from build123d import *

# Parameters (mm, degrees)
RESSALTO_EXTRUS_O1_DEPTH = 20


with BuildPart() as part:
    # Esboço1 → Ressalto-extrusão1 (new body, symmetric)
    with BuildSketch(Plane.XY):
        with BuildLine():
            Line((-40, 0), (40, 0))
            ThreePointArc((40, 0), (47.071067812, 2.928932188), (50, 10))
            Line((50, 10), (50, 110))
            ThreePointArc((50, 110), (51.339745962, 115), (55, 118.660254038))
            Line((55, 118.660254038), (95, 141.754264805))
            ThreePointArc((95, 141.754264805), (98.660254038, 145.414518843), (100, 150.414518843))
            Line((100, 150.414518843), (100, 290))
            ThreePointArc((100, 290), (97.071067812, 297.071067812), (90, 300))
            Line((90, 300), (-90, 300))
            ThreePointArc((-90, 300), (-97.071067812, 297.071067812), (-100, 290))
            Line((-100, 290), (-100, 150.414518843))
            ThreePointArc((-100, 150.414518843), (-98.660254038, 145.414518843), (-95, 141.754264805))
            Line((-95, 141.754264805), (-55, 118.660254038))
            ThreePointArc((-55, 118.660254038), (-51.339745962, 115), (-50, 110))
            Line((-50, 110), (-50, 10))
            ThreePointArc((-50, 10), (-47.071067812, 2.928932188), (-40, 0))
        make_face()
    extrude(amount=RESSALTO_EXTRUS_O1_DEPTH, both=True)


solid = part.part
Could you check a few things on this model? Use its own coordinates, in mm. A direction names the side the tool comes from. Give positions to 0.01 mm unless a question says otherwise; leave off trailing zeros. Order: outer loops, then holes, each group sorted by start corner. A loop starts at its lowest first (then second) coordinate and runs counter-clockwise, first axis right, second up. Notation, with made-up numbers: (-10, 30.5) - (-2, 30.5) arc R28 ccw to (-2, 66.5) - close; hole circle Ø1 at (43, -17.75). An arc over 180 degrees is marked (long way). Return JSON: item names as keys, results as strings. Group by question number.
Q1. Will these pins go through, and if not, where does the flat tip stop? pin 1 Ø8 at (x, z) = (-61.5, -15.5) entering from -Y; pin 2 Ø12 at (y, z) = (40, 9) entering from +X.
Q2. Suppose I cut it at C-C, the plane x = -79. Please give me the cut outline in (y, z).
Q3. Which directions (+Z, -Z, +X, -X, +Y, -Y) give clear straight access to the entire face, cutting with the end or side of a thin tool? Please do faces 1 (the face through (-50, 61, 0)), 2 (the face through (50, 59, 0)), 3 (the face through (-1, 0, 0)).
Q4. Suppose I cut it at B-B, the plane y = 69. Please give me the cut outline in (x, z).
Q5. Please list where these lines run through material, in increasing order: line 1 along X through (y, z) = (18, -8); line 2 along Y through (x, z) = (58.5, 6); line 3 along Y through (x, z) = (57, 6). Write a range as [from, to].
Q6. Suppose I cut it at A-A, the plane z = 4. Please give me the cut outline in (x, y), and give its area (3 significant figures).
Resolved:
{
 "1": {"pin 1": "stops at y = 120.1", "pin 2": "stops at x = 50"},
 "2": {"outline": "(132.52, -20) - (300, -20) - (300, 20) - (132.52, 20) - close"},
 "3": {"face 1": "+Z, -Z, -X, -Y", "face 2": "+Z, -Z, +X, -Y", "face 3": "+Z, -Z, +X, -X, -Y"},
 "4": {"outline": "(-50, -20) - (50, -20) - (50, 20) - (-50, 20) - close"},
 "5": {"line 1": "x = [-50, 50]", "line 2": "y = [120.68, 300]", "line 3": "y = [119.81, 300]"},
 "6": {"outline": "(-100, 150.41) arc R10 ccw to (-95, 141.75) - (-55, 118.66) arc R10 cw to (-50, 110) - (-50, 10) arc R10 ccw to (-40, 0) - (40, 0) arc R10 ccw to (50, 10) - (50, 110) arc R10 cw to (55, 118.66) - (95, 141.75) arc R10 ccw to (100, 150.41) - (100, 290) arc R10 ccw to (90, 300) - (-90, 300) arc R10 ccw to (-100, 290) - close", "area": "46,900 mm2"}
}
